Could you check a few things on this model? Use its own coordinates, in mm. A direction names the side the tool comes from. Coordinates: 2 decimals unless noted, no trailing zeros. Loops run counter-clockwise (first coordinate to the right, second up) from the corner with the lowest first, then second, coordinate; pieces in that order, holes last. Notation, with made-up numbers: M 58,-8.5 L 75,-8.5 A23 ccw 75,13.5 Z; hole C -34,-34 d6. An arc over 180 degrees is marked long. Write each question's results on one line, items separated by ' | '.
```python
from build123d import *

# Parameters (mm, degrees)
BASE_DEPTH          = 417
CHAMFER1_SIZE       = 3
SKETCH3_R           = 1.55
FORCABLECHAIN_DEPTH = 10
SKETCH4_R           = 1.55
GUIDEHOLES_DEPTH    = 418.958131874
SKETCH5_R           = 2
CABLETIEHOLES_DEPTH = 418.958131874


with BuildPart() as part:
    # Sketch1 → Base (new body)
    with BuildSketch(Plane.XY):
        Polygon((0, 0), (20, 0), (20, 1), (1, 1), (1, 20), (0, 20), align=None)
    extrude(amount=BASE_DEPTH)

    # Chamfer1
    chamfer1_edges = [part.edges().sort_by_distance(p)[0] for p in [
        (20, 0.5, 417),
        (0.5, 20, 417),
        (0.5, 20, 0),
        (20, 0.5, 0),
    ]]
    chamfer(chamfer1_edges, length=CHAMFER1_SIZE)

    # Sketch3 → ForCableChain (cut)
    with BuildSketch(Plane(origin=(1, 0, 0), x_dir=(0, 0, -1), z_dir=(1, 0, 0))):
        with Locations(Location((-168, 14.85, 0), (0, 0, 90))):
            Circle(SKETCH3_R)
        with Locations(Location((-160.2, 7.35, 0), (0, 0, 90))):
            Circle(SKETCH3_R)
    extrude(amount=-FORCABLECHAIN_DEPTH, mode=Mode.SUBTRACT)

    # Sketch4 → GuideHoles (cut, through all)
    with BuildSketch(Plane.XZ):
        with Locations(Location((7.25, 10, 0), (0, 0, 270))):
            Circle(SKETCH4_R)
        with Locations(Location((14.75, 16, 0), (0, 0, 270))):
            Circle(SKETCH4_R)
        with Locations(Location((7.25, 401, 0), (0, 0, 270))):
            Circle(SKETCH4_R)
        with Locations(Location((14.75, 407, 0), (0, 0, 270))):
            Circle(SKETCH4_R)
    extrude(amount=-GUIDEHOLES_DEPTH, mode=Mode.SUBTRACT)

    # Sketch5 → CableTieHoles (cut, through all)
    with BuildSketch(Plane.XZ):
        with Locations(Location((11, 25, 0), (0, 0, 270))):
            Circle(SKETCH5_R)
        with Locations(Location((11, 135, 0), (0, 0, 270))):
            Circle(SKETCH5_R)
    extrude(amount=-CABLETIEHOLES_DEPTH, mode=Mode.SUBTRACT)


solid = part.part
```
(1) Please list where these lines run through material, in increasing order: probe 1 along X at (y, z) = (0.55, 407); probe 2 along X at (y, z) = (0.4, 25); probe 3 along Z at (x, y) = (0.5, 7.35). Write a range as from..to.
Reported:
probe 1: x = 0..13.2, 16.3..20 | probe 2: x = 0..9, 13..20 | probe 3: z = 0..158.65, 161.75..417
(2) Imagine slicing it at A-A, the plane z = 123.5. List the corners of the cut face in (x, y) for me.
Reported:
outline: M 0,0 L 20,0 L 20,1 L 1,1 L 1,20 L 0,20 Z
(3) Will these pins go through, and if not, where does the flat tip stop? P1, Ø9.5, axis at y = 13, z = 135.5, coming from the +X side; P2, Ø2, axis at x = 3.5, y = 16.5, coming from the -Z side; P3, Ø8, axis at x = 9, z = 66.5, coming from the +Y side.
Reported:
P1: stops at x = 1 | P2: passes through | P3: stops at y = 1
(4) Which directions (+Z, -Z, +X, -X, +Y, -Y) give clear straight access to the entire face, cutting with the end or side of a thin tool? Please do faces 1 (the flat face through (1, 10, 206)), 2 (the flat face through (10, 0, 206)).
Reported:
face 1: +Z, -Z, +X, +Y | face 2: +Z, -Z, +X, -X, -Y
